Geometry check sheet. Reference: the model listing, model coordinates, mm. Give positions to 0.01 mm unless a question says otherwise; leave off trailing zeros. Order: outer loops, then holes, each group sorted by start corner. A loop starts at its lowest first (then second) coordinate and runs counter-clockwise, first axis right, second up. Notation, with made-up numbers: M 54,-4 L 74,-4 A17 ccw 74,8 Z; hole C -6.75,-3.5 d8. An arc over 180 degrees is marked long. Answer as CSV lines item,"result".
from build123d import *

# Parameters (mm, degrees)
SKETCH1_R           = 3
SKETCH1_R_2         = 1.75
BOSS_EXTRUDE1_DEPTH = 10
MOVE_FACE1_BY       = 5
MOVE_FACE2_BY       = 10


with BuildPart() as part:
    # Sketch1 → Boss-Extrude1 (new body)
    with BuildSketch(Plane(origin=(0, 0, 0), x_dir=(1, 0, 0), z_dir=(0, 1, 0))):
        with Locations(Location((0, 0, 0), (0, 0, 270))):
            Circle(SKETCH1_R)
        with Locations(Location((0, 0, 0), (0, 0, 270))):
            Circle(SKETCH1_R_2, mode=Mode.SUBTRACT)
    extrude(amount=BOSS_EXTRUDE1_DEPTH)

    # Move Face1: a face moved outward by 5.0
    extrude(part.faces().sort_by_distance((0, 0, 2.4))[0], amount=MOVE_FACE1_BY, dir=(0, -1, 0))

    # Move Face2: a face moved inward by 10.0
    extrude(part.faces().sort_by_distance((0, -5, 2.4))[0], amount=MOVE_FACE2_BY, dir=(0, 1, 0), mode=Mode.SUBTRACT)


solid = part.part
(1) Section check C-C on y = 9.3. Enter the section's corners in (x, z).
The answers:
outline,"C 0,0 d6; hole C 0,0 d3.5"
(2) Section check A-A on z = 0. Enter the section's corners in (x, y), then the cut area to 3 significant figures.
The answers:
outline,"M -3,5 L -1.75,5 L -1.75,10 L -3,10 Z; M 1.75,5 L 3,5 L 3,10 L 1.75,10 Z"
area,"12.5 mm2"
(3) Material ranges on line 1 (X direction, y = 8, z = 0); line 2 (Z direction, x = 1.5, y = 9.1); line 3 (Z direction, x = 1.3, y = 8.75), recorded low to high.
The answers:
line 1,"x = -3 to -1.75, 1.75 to 3"
line 2,"z = -2.6 to -0.9, 0.9 to 2.6"
line 3,"z = -2.7 to -1.17, 1.17 to 2.7"
(4) Gauge pin test, flat end, axial feed: P1, Ø1, axis at x = -1.5, y = 7.5, coming from the +Z side. Record the tip position at first contact, or that the pin passes through.
The answers:
P1,"stops at z = 2.83"
(5) Section check B-B on x = 0. Enter the section's corners in (y, z).
The answers:
outline,"M 5,-3 L 10,-3 L 10,-1.75 L 5,-1.75 Z; M 5,1.75 L 10,1.75 L 10,3 L 5,3 Z"
(6) Section check D-D on z = -2.15. Enter the section's corners in (x, y).
The answers:
outline,"M -2.09,5 L 2.09,5 L 2.09,10 L -2.09,10 Z"
(7) Draft check along X on faces 1 (the face through (0.9, 7.54, 2.86)), 2 (the face through (-1.71, 7.46, -0.38)), 3 (the face through (-2, 10, 0)). Enter one of: +X half, -X half, draft (parallel to the pull), parting line (faces both ways), or undercut.
The answers:
face 1,"parting line"
face 2,"undercut"
face 3,"draft"
